Build history of the part. All positions in model axes, mm. Face numbers are marked on the shaded views. A direction names the side the tool comes from. Round coordinates to 2 decimals unless told otherwise and drop trailing zeros. Order: outer loops, then holes, each group sorted by start corner. A loop starts at its lowest first (then second) coordinate and runs counter-clockwise, first axis right, second up. Notation, with made-up numbers: (50.25, 41) - (101.25, 41) arc R17 ccw to (101.25, 73) - close; hole circle Ø6 at (7.25, -14.75). An arc over 180 degrees is marked (long way). Write each question's results on one line, items separated by ' | '. Start each with the question number.
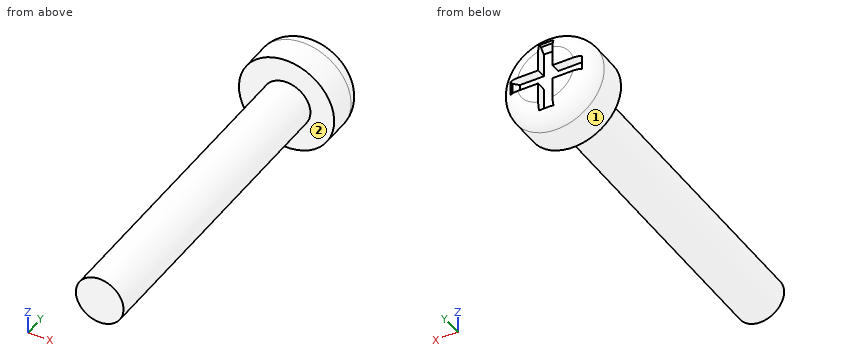
```python
from build123d import *

# Parameters (mm, degrees)
SKETCH1_R           = 2
BOSS_EXTRUDE1_DEPTH = 2
FILLET1_R           = 0.8
SKETCH2_W           = 0.6
SKETCH2_H           = 0.6
CUT_EXTRUDE1_DEPTH  = 0.4
CHAMFER1_SIZE       = 0.2
SKETCH3_R           = 1
BOSS_EXTRUDE2_DEPTH = 13.3


with BuildPart() as part:
    # Sketch1 → Boss-Extrude1 (new body)
    with BuildSketch(Plane(origin=(0, 0, 0), x_dir=(1, 0, 0), z_dir=(0, 1, 0))):
        with Locations(Location((0, 0, 0), (0, 0, 270))):
            Circle(SKETCH1_R)
    extrude(amount=BOSS_EXTRUDE1_DEPTH)

    # Fillet1
    fillet1_edges = [part.edges().sort_by_distance(p)[0] for p in [
        (0, 2, -2),
    ]]
    fillet(fillet1_edges, radius=FILLET1_R)

    # Sketch2 → Cut-Extrude1 (cut)
    with BuildSketch(Plane(origin=(0, 2, 0), x_dir=(1, 0, 0), z_dir=(0, 1, 0))):
        with BuildLine():
            Line((-0.3, 0.3), (-1.161895004, 0.3))
            ThreePointArc((-1.161895004, 0.3), (-1.2, 0), (-1.161895004, -0.3))
            Line((-1.161895004, -0.3), (-0.3, -0.3))
            Line((-0.3, -0.3), (-0.3, 0.3))
        make_face()
        with BuildLine():
            Line((-0.3, 1.161895004), (-0.3, 0.3))
            Line((-0.3, 0.3), (0.3, 0.3))
            Line((0.3, 0.3), (0.3, 1.161895004))
            ThreePointArc((0.3, 1.161895004), (0, 1.2), (-0.3, 1.161895004))
        make_face()
        with BuildLine():
            Line((-1.161895004, 0.3), (-1.5, 0.3))
            Line((-1.5, 0.3), (-1.5, -0.3))
            Line((-1.5, -0.3), (-1.161895004, -0.3))
            ThreePointArc((-1.161895004, -0.3), (-1.2, 0), (-1.161895004, 0.3))
        make_face()
        with BuildLine():
            Line((-0.3, 1.5), (-0.3, 1.161895004))
            ThreePointArc((-0.3, 1.161895004), (0, 1.2), (0.3, 1.161895004))
            Line((0.3, 1.161895004), (0.3, 1.5))
            Line((0.3, 1.5), (-0.3, 1.5))
        make_face()
        with BuildLine():
            Line((1.161895004, 0.3), (0.3, 0.3))
            Line((0.3, 0.3), (0.3, -0.3))
            Line((0.3, -0.3), (1.161895004, -0.3))
            ThreePointArc((1.161895004, -0.3), (1.190435636, -0.151205151), (1.2, 0))
            ThreePointArc((1.2, 0), (1.190435636, 0.151205151), (1.161895004, 0.3))
        make_face()
        with BuildLine():
            Line((1.5, 0.3), (1.161895004, 0.3))
            ThreePointArc((1.161895004, 0.3), (1.190435636, 0.151205151), (1.2, 0))
            ThreePointArc((1.2, 0), (1.190435636, -0.151205151), (1.161895004, -0.3))
            Line((1.161895004, -0.3), (1.5, -0.3))
            Line((1.5, -0.3), (1.5, 0.3))
        make_face()
        Rectangle(SKETCH2_W, SKETCH2_H)
        with BuildLine():
            Line((0.3, -0.3), (-0.3, -0.3))
            Line((-0.3, -0.3), (-0.3, -1.161895004))
            ThreePointArc((-0.3, -1.161895004), (0, -1.2), (0.3, -1.161895004))
            Line((0.3, -1.161895004), (0.3, -0.3))
        make_face()
        with BuildLine():
            ThreePointArc((0.3, -1.161895004), (0, -1.2), (-0.3, -1.161895004))
            Line((-0.3, -1.161895004), (-0.3, -1.5))
            Line((-0.3, -1.5), (0.3, -1.5))
            Line((0.3, -1.5), (0.3, -1.161895004))
        make_face()
    extrude(amount=-CUT_EXTRUDE1_DEPTH, mode=Mode.SUBTRACT)

    # Chamfer1
    chamfer1_edges = [part.edges().sort_by_distance(p)[0] for p in [
        (-1.5, 1.6, 0),
        (0, 1.6, 1.5),
        (0, 1.6, -1.5),
        (1.5, 1.6, 0),
    ]]
    chamfer(chamfer1_edges, length=CHAMFER1_SIZE)

    # Sketch3 → Boss-Extrude2 (add)
    with BuildSketch(Plane.XZ):
        with Locations(Location((0, 0, 0), (0, 0, 270))):
            Circle(SKETCH3_R)
    extrude(amount=BOSS_EXTRUDE2_DEPTH)


solid = part.part
```
1. 3-axis set-ups, long thin cutter, end or side, ignore diameter. For the marked faces 1 and 2: which of +Z, -Z, +X, -X, +Y, -Y reach the whole face in a straight line?
2. Cut at C-C (y = -0.75). List the corners of the cut face in (x, z).
3. Flat gauge pin, fed straight in: pin 1 Ø2 at (x, y) = (-1, -10) entering from -Z. Where does the tip first touch, or does it go through?
4. Cut at B-B (z = 0). List the corners of the cut face in (x, y).
5. Cut at A-A (x = 0). List the corners of the cut face in (y, z).
6. Wall check: line 1 (Y direction, x = 0.05, z = 0); line 2 (Y direction, x = -0.25, z = 1.15); line 3 (Z direction, x = 0.95, y = 1.25). Give the ranges that are in metal, low to high. Write a range as from..to.
A:
1) face 1: +Y, -Y | face 2: -Y
2) outline: circle Ø2 at (0, 0)
3) pin 1: stops at z = -1
4) outline: (-2, 0) - (-1, 0) - (-1, -13.3) - (1, -13.3) - (1, 0) - (2, 0) - (2, 1.2) arc R0.8 ccw to (1.5, 1.94) - (1.5, 1.8) - (1.3, 1.6) - (-1.3, 1.6) - (-1.5, 1.8) - (-1.5, 1.94) arc R0.8 ccw to (-2, 1.2) - close
5) outline: (-13.3, -1) - (0, -1) - (0, -2) - (1.2, -2) arc R0.8 ccw to (1.94, -1.5) - (1.8, -1.5) - (1.6, -1.3) - (1.6, 1.3) - (1.8, 1.5) - (1.94, 1.5) arc R0.8 ccw to (1.2, 2) - (0, 2) - (0, 1) - (-13.3, 1) - close
6) line 1: y = -13.3..1.6 | line 2: y = 0..1.6 | line 3: z = -1.76..1.76
